from build123d import *

# Parameters (mm, degrees)
F0_W           = 24
F0_H           = 11.6
F1_DEPTH       = 3
F3_D           = 3
F3_CBORE_D     = 6.5
F3_CBORE_DEPTH = 1.5
F4_DEPTH       = 28
F7_R           = 4
F8_R           = 9.25
F9_DEPTH       = 25
F10_DEPTH      = 5
F11_DEPTH      = 2
F2_W           = 2
F2_H           = 8.1
F12_REACH      = 36.3442607534
F5_W           = 2
F5_H           = 8.1
F13_REACH      = 36.3442607534
F14_SIZE       = 1
F15_R          = 2
F17_DEPTH      = 25


# Not quite as in the source:
# - a feature names something its author has since deleted; it is built from what else it names


with BuildPart() as f1:
    # F0 (on Front) → F1 (new body)
    with BuildSketch(Plane.XZ):
        with Locations((12, 5.8)):
            Rectangle(F0_W, F0_H)
    extrude(amount=F1_DEPTH)

    # F3 (through all)
    with Locations(Plane.XZ.offset(3)):
        with Locations((6.5, 7.1), (17.5, 7.1)):
            CounterBoreHole(F3_D / 2, F3_CBORE_D / 2, F3_CBORE_DEPTH)

    # F2 (on face) → F4 (join)
    with BuildSketch(Plane.XZ.offset(3)):
        Polygon((0, 3.5), (0, 0), (24, 0), (24, 3.5), (22, 3.5), (2, 3.5), align=None)
    extrude(amount=F4_DEPTH)

    # F7
    f7_edges = [f1.edges().sort_by_distance(p)[0] for p in [
        (24, -31, 1.75),
        (0, -31, 1.75),
    ]]
    fillet(f7_edges, radius=F7_R)

    # F8 (on face) → F9 (cut)
    with BuildSketch(Plane(origin=(0, 0, 0), x_dir=(1, 0, 0), z_dir=(0, 0, -1))):
        with Locations((12, 16.9718765144)):
            Circle(F8_R)
    extrude(amount=-F9_DEPTH, mode=Mode.SUBTRACT)

    # F10 (add): a face of the model
    f10_faces = [f1.faces().sort_by_distance(p)[0] for p in [
        (0.3920459157, -13.5, 0),
    ]]
    extrude(f10_faces, amount=F10_DEPTH)

    # F6 (on face) → F11 (cut)
    with BuildSketch(Plane.XY.offset(3.5)):
        Polygon((24, -24.0155497985), (24, -9.9282032303), (12, -3), (0, -9.9282032303), (0, -24.0155497985), (12, -30.9437530288), align=None)
    extrude(amount=-F11_DEPTH, mode=Mode.SUBTRACT)

    f12_end = Plane(origin=(6, -6.4641016151, 2.5), x_dir=(-0.8660254038, -0.5, 0), z_dir=(0.5, -0.8660254038, 0))
    # F2 (on face) → F12 (join, up to a plane its end follows)
    with BuildSketch(Plane.XZ.offset(3)):
        with Locations((1, 7.55)):
            Rectangle(F2_W, F2_H)
    f12_long = extrude(amount=F12_REACH, mode=Mode.PRIVATE)
    add(split(f12_long, bisect_by=f12_end, keep=Keep.BOTTOM, mode=Mode.PRIVATE))

    f13_end = Plane(origin=(18, -6.4641016151, 2.5), x_dir=(-0.8660254038, 0.5, 0), z_dir=(-0.5, -0.8660254038, 0))
    # F5 (on face) → F13 (join, up to a plane its end follows)
    with BuildSketch(Plane.XZ.offset(3)):
        with Locations((23, 7.55)):
            Rectangle(F5_W, F5_H)
    f13_long = extrude(amount=F13_REACH, mode=Mode.PRIVATE)
    add(split(f13_long, bisect_by=f13_end, keep=Keep.BOTTOM, mode=Mode.PRIVATE))

    # F14
    f14_edges = [f1.edges().sort_by_distance(p)[0] for p in [
        (12, 0, -5),
    ]]
    chamfer(f14_edges, length=F14_SIZE)

    # F15
    f15_edges = [f1.edges().sort_by_distance(p)[0] for p in [
        (24, -4.964102, 11.6),
        (0, -4.964102, 11.6),
    ]]
    fillet(f15_edges, radius=F15_R)

    # F16 (on face) → F17 (cut)
    with BuildSketch(Plane.YZ.offset(24)):
        Polygon((-9.9282032303, 11.6), (-9.9282032303, 1.5), (-3, 11.6), align=None)
    extrude(amount=-F17_DEPTH, mode=Mode.SUBTRACT)


solid = f1.part
Input: part model. Units: mm. Frame: model coordinates. A direction names the side the tool comes from. Round coordinates to 2 decimals unless told otherwise and drop trailing zeros. Order: outer loops, then holes, each group sorted by start corner. A loop starts at its lowest first (then second) coordinate and runs counter-clockwise, first axis right, second up.
1. Cut plane D-D, the plane x = 15. Output: boundary loops of the cut face in (y, z).
The answers:
outline: (-31, -5) - (-25.72, -5) - (-25.72, 1.5) - (-29.21, 1.5) - (-29.21, 3.5) - (-31, 3.5) - close; (-8.22, -5) - (-1, -5) - (0, -4) - (0, 11.6) - (-3, 11.6) - (-3, 9.18) - (-1.5, 9.18) - (-1.5, 5.02) - (-3, 5.02) - (-3, 3.5) - (-4.73, 3.5) - (-4.73, 1.5) - (-8.22, 1.5) - close
2. Cut plane A-A, the plane x = 7.5. Output: boundary loops of the cut face in (y, z).
The answers:
outline: (-31, -5) - (-25.05, -5) - (-25.05, 1.5) - (-28.35, 1.5) - (-28.35, 3.5) - (-31, 3.5) - close; (-8.89, -5) - (-1, -5) - (0, -4) - (0, 5.98) - (-1.5, 5.98) - (-1.5, 4.01) - (-3, 4.01) - (-3, 3.5) - (-5.6, 3.5) - (-5.6, 1.5) - (-8.89, 1.5) - close; (-3, 10.19) - (-1.5, 10.19) - (-1.5, 8.22) - (0, 8.22) - (0, 11.6) - (-3, 11.6) - close
3. Cut plane B-B, the plane z = 7.1. Output: boundary loops of the cut face in (x, y), then the cut area to 3 significant figures.
The answers:
outline: (0, -6.09) - (2, -6.09) - (2, -3) - (3.25, -3) - (3.25, -1.5) - (5, -1.5) - (5, 0) - (0, 0) - close; (8, -1.5) - (9.75, -1.5) - (9.75, -3) - (14.25, -3) - (14.25, -1.5) - (16, -1.5) - (16, 0) - (8, 0) - close; (19, -1.5) - (20.75, -1.5) - (20.75, -3) - (22, -3) - (22, -6.09) - (24, -6.09) - (24, 0) - (19, 0) - close
area: 55.8 mm2
4. Mould query, pull axis X, two halves, no side actions, for faces 1 (the face through (5.916, -27.431, 2.514)), 2 (the face through (12, -3, 8)), 3 (the face through (0.57, -1.67, 11)), 4 (the face through (0.9, -6.5, 6.5)). Classes: released by +X, released by -X, zero draft, split by the parting line, or undercut.
The answers:
face 1: undercut
face 2: undercut
face 3: released by -X
face 4: zero draft
5. Material intervals for line 1 (Y direction, x = 12, z = -2); line 2 (Y direction, x = 6, z = -0.5); line 3 (Y direction, x = 2.75, z = 6.25), sorted ascending.
The answers:
line 1: y = -31 to -26.22, -7.72 to 0
line 2: y = -31 to -24.01, -9.93 to 0
line 3: y = -3 to 0
6. Pin query (flat end, axial travel): P1, Ø4, axis at x = 17.5, z = 7.1, coming from the -Y side; P2, Ø1, axis at x = 12.5, y = -8, coming from the +Z side; P3, Ø4, axis at x = 9.5, z = 6, coming from the -Y side. Return the tip coordinate at first contact, or that it passes through.
The answers:
P1: stops at y = -1.5
P2: stops at z = 1.5
P3: stops at y = -3
7. Set-up query: faces 5 (the face through (6, -5, 3.5)), 6 (the face through (13.72, -26.22, 1.5)), 7 (the face through (23.1, -6.5, 6.5)), 8 (the face through (14.253, -2.26, 7.243)). Return all of +Z, -Z, +X, -X, +Y, -Y with unobstructed straight access to the full face (end or side cutting, diameter ignored); none if empty.
The answers:
face 5: +Z, -Y
face 6: +Z
face 7: +Z, +X, -X
face 8: -Y
8. Cut plane C-C, the plane y = -13. Output: boundary loops of the cut face in (x, z).
The answers:
outline: (0, -5) - (3.65, -5) - (3.65, 1.5) - (0, 1.5) - close; (20.35, -5) - (24, -5) - (24, 1.5) - (20.35, 1.5) - close
